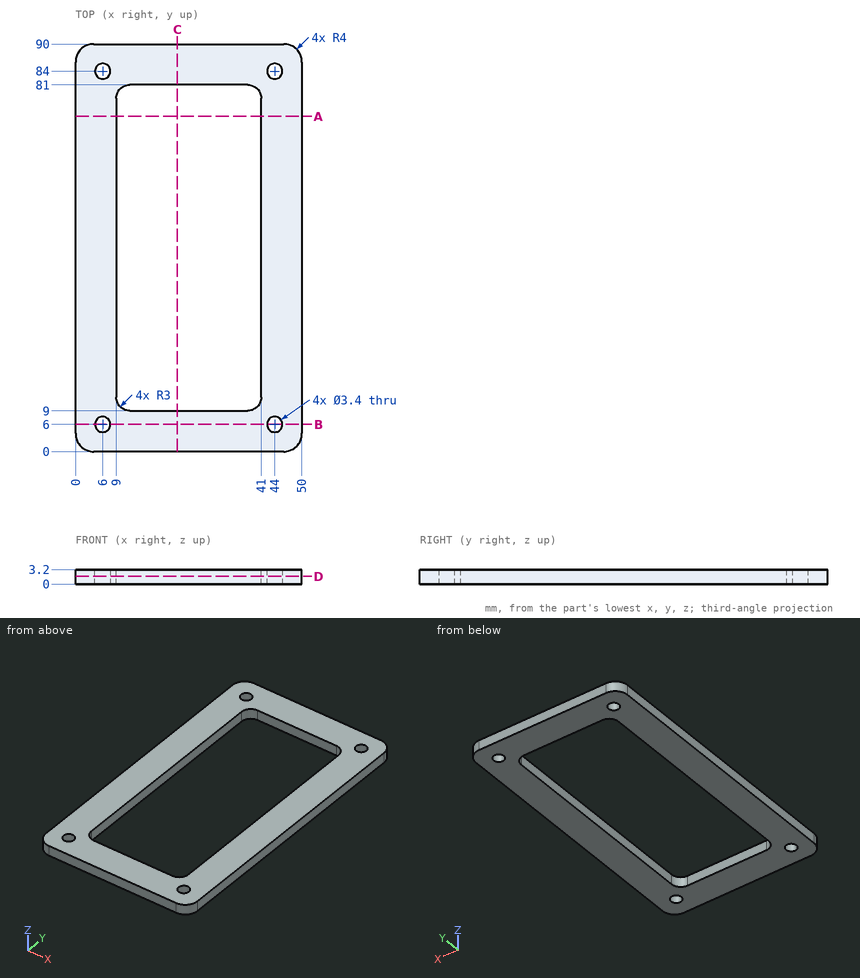
Geometry: see drawing. Coordinates: mm, zero at the bounding-box minimum. Round coordinates to 2 decimals unless told otherwise and drop trailing zeros. Order: outer loops, then holes, each group sorted by start corner. A loop starts at its lowest first (then second) coordinate and runs counter-clockwise, first axis right, second up. Notation, with made-up numbers: (-4.5, -37.5) - (19.5, -37.5) arc R20 cw to (19.5, -27.5) - close; hole circle Ø6 at (11, 20.5). An arc over 180 degrees is marked (long way). One line per question, with ' | ' between items. Start each with the question number.
1) Cut plane C-C, the plane x = 22.5. Return the cut outline in (y, z), then the cut area to 3 significant figures.
2) Ray query, probe 1 along X at (y, z) = (84, 1.85); probe 2 along Y at (x, z) = (6, 2.5); probe 3 along Y at (x, z) = (22, 2.3). Return the intervals inside material, ascending.
3) Cut plane A-A, the plane y = 74. Return the cut outline in (x, z).
4) Cut plane B-B, the plane y = 6. Return the cut outline in (x, z), then the cut area to 3 significant figures.
5) Cut plane D-D, the plane z = 1.7. Return the cut outline in (x, y), then the cut area to 3 significant figures.
Worked out:
1) outline: (0, 0) - (9, 0) - (9, 3.2) - (0, 3.2) - close; (81, 0) - (90, 0) - (90, 3.2) - (81, 3.2) - close | area: 57.6 mm^2
2) probe 1: x = 0 to 4.3, 7.7 to 42.3, 45.7 to 50 | probe 2: y = 0 to 4.3, 7.7 to 82.3, 85.7 to 90 | probe 3: y = 0 to 9, 81 to 90
3) outline: (0, 0) - (9, 0) - (9, 3.2) - (0, 3.2) - close; (41, 0) - (50, 0) - (50, 3.2) - (41, 3.2) - close
4) outline: (0, 0) - (4.3, 0) - (4.3, 3.2) - (0, 3.2) - close; (7.7, 0) - (42.3, 0) - (42.3, 3.2) - (7.7, 3.2) - close; (45.7, 0) - (50, 0) - (50, 3.2) - (45.7, 3.2) - close | area: 138 mm^2
5) outline: (0, 4) arc R4 ccw to (4, 0) - (46, 0) arc R4 ccw to (50, 4) - (50, 86) arc R4 ccw to (46, 90) - (4, 90) arc R4 ccw to (0, 86) - close; hole circle Ø3.4 at (6, 6); hole circle Ø3.4 at (6, 84); hole (9, 12) arc R3 ccw to (12, 9) - (38, 9) arc R3 ccw to (41, 12) - (41, 78) arc R3 ccw to (38, 81) - (12, 81) arc R3 ccw to (9, 78) - close; hole circle Ø3.4 at (44, 6); hole circle Ø3.4 at (44, 84) | area: 2,150 mm^2
